Part print with two shaded views. Sizes in mm from the minimum x, y, z corner. Round coordinates to 2 decimals unless told otherwise and drop trailing zeros. Write each loop counter-clockwise with the first axis right and the second up, starting at its lowest first coordinate (ties: lowest second). Pieces come first, ordered by that corner, then holes. Notation, with made-up numbers: (37.25, 89.5) -> (55.25, 89.5) arc R9 cw to (55.25, 94.5) -> close; hole circle Ø9 at (61, 42). An arc over 180 degrees is marked (long way). Return JSON: item names as keys, results as strings. Group by question number.
(1) Drill centre lines: L1, parallel to Z at x = 50, y = 6.5; L2, parallel to X at y = 9.75, z = 46.5; L3, parallel to Z at x = 45.5, y = 11.25. Where is each one in solid material? Low to high. Write a range as from..to.
(2) Saw through at B-B (z = 50). List the corners of the cut face in (x, y), plus the area to 3 significant figures.
(3) Drop a flat-ended pin along its axis: pin 1 Ø2 at (x, z) = (52, 50) entering from -Y. Give the stop position or say it passes through.
(4) Saw through at A-A (x = 50). List the corners of the cut face in (y, z).
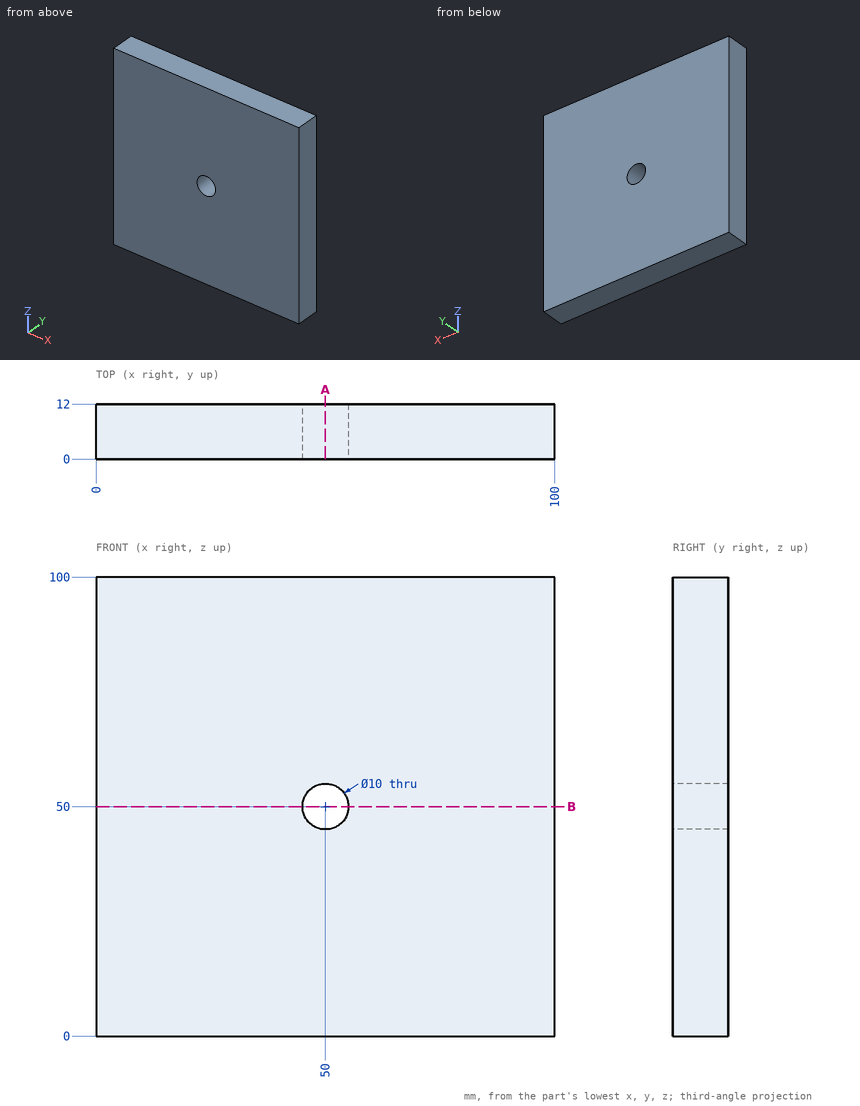
Computed values:
{
 "1": {"L1": "0..45, 55..100", "L2": "0..46.43, 53.57..100", "L3": "0..47.82, 52.18..100"},
 "2": {"outline": "(0, 0) -> (45, 0) -> (45, 12) -> (0, 12) -> close; (55, 0) -> (100, 0) -> (100, 12) -> (55, 12) -> close", "area": "1,080 mm2"},
 "3": {"pin 1": "through"},
 "4": {"outline": "(0, 0) -> (12, 0) -> (12, 45) -> (0, 45) -> close; (0, 55) -> (12, 55) -> (12, 100) -> (0, 100) -> close"}
}
